Part print with two shaded views. Sizes in mm from the minimum x, y, z corner. A direction names the side the tool comes from. Round coordinates to 2 decimals unless told otherwise and drop trailing zeros. Write each loop counter-clockwise with the first axis right and the second up, starting at its lowest first coordinate (ties: lowest second). Pieces come first, ordered by that corner, then holes. Notation, with made-up numbers: M -30,31 L -8,31 A31 ccw -8,56 Z; hole C 26,87.25 d11. An arc over 180 degrees is marked long. One line per question, with ' | ' between items. Start each with the question number.
1) Saw through at C-C (y = 2.65). List the corners of the cut face in (x, z).
2) Saw through at A-A (z = 11.5). List the corners of the cut face in (x, y) (3 decimals).
3) Drop flat-ended pins along their axis: pin 1 Ø1.2 at (x, y) = (2.5, 2) entering from -Z; pin 2 Ø1.5 at (y, z) = (3.5, 18) entering from -X. Give the stop position or say it passes through.
4) Mould opens along X. For the marked faces 3, 4 and 5 say: pulls with the +X half, pulls with the -X half, needs draft (parallel to the pull), parting line crosses it, or undercut.
5) Saw through at B-B (x = 2.8). List the corners of the cut face in (y, z) (1 decimal).
6) Wall check: probe 1 along Y at (x, z) = (2.5, 6.5) (3 decimals); probe 2 along X at (y, z) = (1.85, 16.25); probe 3 along Z at (x, y) = (3.3, 0.4). Give the ranges that are in metal, low to high. Write a range as [from, to].
7) Saw through at D-D (z = 19.25). List the corners of the cut face in (x, y) (3 decimals), plus the area to 3 significant figures.
8) Tool access for the marked faces 1 and 2: list every direction of +Z, -Z, +X, -X, +Y, -Y with a clear straight run to the whole face (end or side of a thin tool).
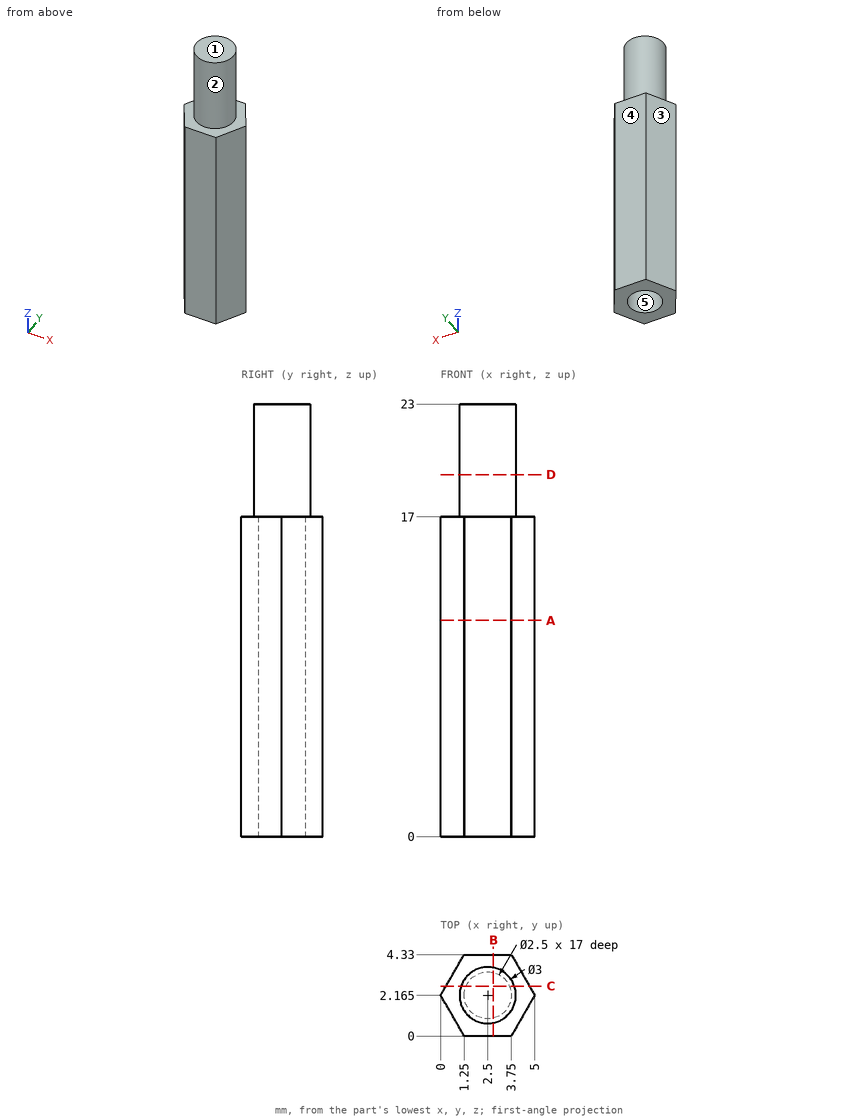
Answer key:
1) outline: M 0.28,0 L 1.35,0 L 1.35,17 L 3.65,17 L 3.65,0 L 4.72,0 L 4.72,17 L 3.92,17 L 3.92,23 L 1.08,23 L 1.08,17 L 0.28,17 Z
2) outline: M 0,2.165 L 1.25,0 L 3.75,0 L 5,2.165 L 3.75,4.33 L 1.25,4.33 Z; hole C 2.5,2.165 d2.5
3) pin 1: stops at z = 17 | pin 2: stops at x = 1.12
4) face 3: pulls with the -X half | face 4: needs draft | face 5: undercut
5) outline: M 0,0 L 1,0 L 1,17 L 3.4,17 L 3.4,0 L 4.3,0 L 4.3,17 L 3.6,17 L 3.6,23 L 0.7,23 L 0.7,17 L 0,17 Z
6) probe 1: y = [0, 0.915], [3.415, 4.33] | probe 2: x = [0.18, 1.29], [3.71, 4.82] | probe 3: z = [0, 17]
7) outline: C 2.5,2.165 d3 | area: 7.07 mm2
8) face 1: +Z, +X, -X, +Y, -Y | face 2: +Z
